Can you work these out from the model? Positions are in its coordinate system, mm. Face numbers are marked on the shaded views. A direction names the side the tool comes from. Give positions to 0.01 mm unless a question says otherwise; leave off trailing zeros. Order: outer loops, then holes, each group sorted by start corner. A loop starts at its lowest first (then second) coordinate and runs counter-clockwise, first axis right, second up. Notation, with made-up numbers: M 54.5,85 L 68.5,85 A11 ccw 68.5,90 Z; hole C 57,34 d8. An arc over 180 degrees is marked long. Write each question's results on one line, items separated by ' | '.
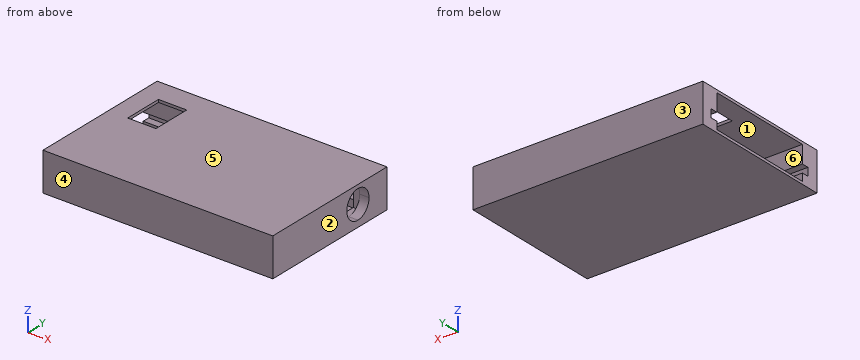
from build123d import *

# Parameters (mm, degrees)
F1_DEPTH      = 6
F1_DEPTH_BACK = 3.5
F2_W          = 1.75
F2_H          = 2
F2_W_2        = 27
F2_H_2        = 1.8599129291
F2_H_3        = 4.3400870709
F3_DEPTH      = 53.001
F4_W          = 7
F4_H          = 9.7
F5_DEPTH      = 0.6599129291
F6_W          = 36
F6_H          = 9.5
F7_DEPTH      = 3.9
F8_DEPTH      = 1.6


with BuildPart() as f1:
    # F0 (on Top) → F1 (new body, two sides)
    with BuildSketch(Plane.XY) as f1_sk:
        Polygon((23.0564765632, 14.9109546933), (-26.9435234368, 14.9109546933), (-26.9435234368, -4.6890453067), (-26.9435234368, -11.6890453067), (-26.9435234368, -15.0890453067), (23.0564765632, -15.0890453067), align=None)
        Polygon((-26.9435234368, 17.9109546933), (-26.9435234368, 14.9109546933), (23.0564765632, 14.9109546933), (23.0564765632, -15.0890453067), (-26.9435234368, -15.0890453067), (-26.9435234368, -18.0890453067), (26.0564765632, -18.0890453067), (26.0564765632, 17.9109546933), align=None)
    extrude(amount=F1_DEPTH)
    extrude(f1_sk.sketch, amount=-F1_DEPTH_BACK)

    # F2 (on face) → F3 (cut, through all)
    with BuildSketch(Plane(origin=(-26.9435234368, 0, 0), x_dir=(0, -1, 0), z_dir=(-1, 0, 0))):
        with Locations((14.375, 0)):
            Rectangle(F2_W, F2_H)
        with Locations((0, -1.9299564646)):
            Rectangle(F2_W_2, F2_H_2)
        with Locations((-14.375, 0)):
            Rectangle(F2_W, F2_H)
        Rectangle(F2_W_2, F2_H)
        with Locations((0, 3.1700435354)):
            Rectangle(F2_W_2, F2_H_3)
    extrude(amount=-F3_DEPTH, mode=Mode.SUBTRACT)

    # F4 (on face) → F5 (cut, through all)
    with BuildSketch(Plane.XY.offset(6)):
        with Locations((-18.6190935215, 7.3109546933)):
            Rectangle(F4_W, F4_H)
    extrude(amount=-F5_DEPTH, mode=Mode.SUBTRACT)

    # F6 (on face) → F7 (join)
    with BuildSketch(Plane.YZ.offset(26.0564765632)):
        with Locations((-0.0890453067, 1.25)):
            Rectangle(F6_W, F6_H)
        Polygon((-15.25, -1), (-15.25, 1), (-13.5, 1), (-13.5, 5.3400870709), (13.5, 5.3400870709), (13.5, 1), (15.25, 1), (15.25, -1), (13.5, -1), (13.5, -2.8599129291), (-13.5, -2.8599129291), (-13.5, -1), align=None, mode=Mode.SUBTRACT)
        Polygon((-13.5, 1), (-15.25, 1), (-15.25, -1), (-13.5, -1), (-13.5, -2.8599129291), (13.5, -2.8599129291), (13.5, -1), (15.25, -1), (15.25, 1), (13.5, 1), (13.5, 5.3400870709), (-13.5, 5.3400870709), align=None)
        Polygon((5.25, 1.6), (5.25, 5.1), (8.75, 5.1), (12.25, 5.1), (12.25, 1.6), (12.25, -1.9), (8.75, -1.9), (5.25, -1.9), align=None, mode=Mode.SUBTRACT)
        with BuildLine():
            Line((8.75, 5.1), (5.25, 5.1))
            Line((5.25, 5.1), (5.25, 1.6))
            ThreePointArc((5.25, 1.6), (6.2751262658, 4.0748737342), (8.75, 5.1))
        make_face()
        with BuildLine():
            Line((12.25, 5.1), (8.75, 5.1))
            ThreePointArc((8.75, 5.1), (11.2248737342, 4.0748737342), (12.25, 1.6))
            Line((12.25, 1.6), (12.25, 5.1))
        make_face()
        with BuildLine():
            Line((12.25, -1.9), (12.25, 1.6))
            ThreePointArc((12.25, 1.6), (11.2248737342, -0.8748737342), (8.75, -1.9))
            Line((8.75, -1.9), (12.25, -1.9))
        make_face()
        with BuildLine():
            ThreePointArc((8.75, -1.9), (6.2751262658, -0.8748737342), (5.25, 1.6))
            Line((5.25, 1.6), (5.25, -1.9))
            Line((5.25, -1.9), (8.75, -1.9))
        make_face()
    extrude(amount=F7_DEPTH)

    # F6 (on face) → F8 (cut)
    with BuildSketch(Plane.YZ.offset(26.0564765632)):
        with BuildLine():
            Line((8.75, 5.1), (5.25, 5.1))
            Line((5.25, 5.1), (5.25, 1.6))
            ThreePointArc((5.25, 1.6), (6.2751262658, 4.0748737342), (8.75, 5.1))
        make_face()
        with BuildLine():
            Line((12.25, 5.1), (8.75, 5.1))
            ThreePointArc((8.75, 5.1), (11.2248737342, 4.0748737342), (12.25, 1.6))
            Line((12.25, 1.6), (12.25, 5.1))
        make_face()
        with BuildLine():
            Line((12.25, -1.9), (12.25, 1.6))
            ThreePointArc((12.25, 1.6), (11.2248737342, -0.8748737342), (8.75, -1.9))
            Line((8.75, -1.9), (12.25, -1.9))
        make_face()
        with BuildLine():
            ThreePointArc((8.75, -1.9), (6.2751262658, -0.8748737342), (5.25, 1.6))
            Line((5.25, 1.6), (5.25, -1.9))
            Line((5.25, -1.9), (8.75, -1.9))
        make_face()
    extrude(amount=F8_DEPTH, mode=Mode.SUBTRACT)


solid = f1.part
(1) I need wall thicknesses on L1, parallel to Y at x = -14.5, z = 3.5; L2, parallel to Y at x = -10, z = -0.75; L3, parallel to Z at x = 26, y = -0.5. Which ranges of each line are inside material? Lowest first, please. Write a range as from..to.
Data:
L1: y = -18.09..-13.5, 13.5..17.91 | L2: y = -18.09..-15.25, 15.25..17.91 | L3: z = -3.5..-2.86, 5.34..6
(2) Will this pin go through, and if not, where does the flat tip stop? P1, Ø1, axis at y = 6.5, z = 4, coming from the -X side.
Data:
P1: stops at x = 27.66
(3) Imagine slicing it at B-B, the plane x = 27. Write out the boundary of the cut face in (y, z).
Data:
outline: M -18.09,-3.5 L 17.91,-3.5 L 17.91,6 L -18.09,6 Z; hole M 5.25,-1.9 L 12.25,-1.9 L 12.25,5.1 L 5.25,5.1 Z
(4) Imagine slicing it at C-C, the plane y = 9.5. Write out the boundary of the cut face in (x, z), plus the area to 3 significant figures.
Data:
outline: M -26.94,-3.5 L 29.96,-3.5 L 29.96,-1.82 L 27.66,-1.82 L 27.66,-1.9 L 26.06,-1.9 L 26.06,-2.86 L -26.94,-2.86 Z; M -26.94,5.34 L -22.12,5.34 L -22.12,6 L -26.94,6 Z; M -15.12,5.34 L 26.06,5.34 L 26.06,5.1 L 27.66,5.1 L 27.66,5.02 L 29.96,5.02 L 29.96,6 L -15.12,6 Z | area: 74.4 mm2
(5) For the marked faces 5 and 6, which set-ups out of +Z, -Z, +X, -X, +Y, -Y let a thin tool reach every point of the face, with its end or its side?
Data:
face 5: +Z, +X, -X, +Y, -Y | face 6: -X
(6) We'd pull the mould along Y, two halves only. Please class the marked faces 1, 2, 3 and 4: +Y half, -Y half, draft (parallel to the pull), parting line (faces both ways), or undercut.
Data:
face 1: undercut | face 2: draft | face 3: +Y half | face 4: -Y half
(7) Imagine slicing it at D-D, the plane y = -3.5. Write out the boundary of the cut face in (x, z).
Data:
outline: M -26.94,-3.5 L 29.96,-3.5 L 29.96,6 L -26.94,6 L -26.94,5.34 L 26.06,5.34 L 26.06,-2.86 L -26.94,-2.86 Z
(8) Imagine slicing it at A-A, the plane z = -0.25. Write out the boundary of the cut face in (x, y), plus the area to 3 significant figures.
Data:
outline: M -26.94,-18.09 L 29.96,-18.09 L 29.96,5.78 L 27.66,5.78 L 27.66,5.25 L 26.06,5.25 L 26.06,-15.25 L -26.94,-15.25 Z; M -26.94,15.25 L 26.06,15.25 L 26.06,12.25 L 27.66,12.25 L 27.66,11.72 L 29.96,11.72 L 29.96,17.91 L -26.94,17.91 Z | area: 407 mm2
